from build123d import *

# Parameters (mm, degrees)
BOSS_EXTRU_1_DEPTH = 22
ESQUISSE3_W        = 22
ESQUISSE3_H        = 178
BOSS_EXTRU_2_DEPTH = 1000


with BuildPart() as part:
    # Esquisse2 → Boss.-Extru.1 (new body)
    with BuildSketch(Plane(origin=(0, 0, 0), x_dir=(1, 0, 0), z_dir=(0, 1, 0))):
        Polygon((-200, 0), (0, 0), (0, 200), (-200, 200), (-200, 105), (-100, 105), (-100, 95), (-200, 95), align=None)
    boss_extru_1 = extrude(amount=BOSS_EXTRU_1_DEPTH)

    # Symétrie1: Boss.-Extru.1 across plane
    add(boss_extru_1.mirror(Plane(origin=(0, 22, 0), x_dir=(0, 0, 1), z_dir=(-1, 0, 0))))

    # Esquisse3 → Boss.-Extru.2 (add)
    with BuildSketch(Plane(origin=(0, 22, 0), x_dir=(1, 0, 0), z_dir=(0, 1, 0))):
        Polygon((70, 200), (-70, 200), (-70, 178), (-11, 178), (11, 178), (70, 178), align=None)
        with Locations((0, 89)):
            Rectangle(ESQUISSE3_W, ESQUISSE3_H)
    extrude(amount=-BOSS_EXTRU_2_DEPTH)


solid = part.part
Part model, mm, in its own coordinate system. A direction names the side the tool comes from. Coordinates: 2 decimals unless noted, no trailing zeros. Order: outer loops, then holes, each group sorted by start corner. A loop starts at its lowest first (then second) coordinate and runs counter-clockwise, first axis right, second up.
(1) Slice it at D-D, the plane x = 54. Write the cut outline in (y, z).
Check sheet entries:
outline: (-978, -200) - (22, -200) - (22, 0) - (0, 0) - (0, -178) - (-978, -178) - close
(2) Probe L1, parallel to Z at x = -19, y = -60.5; L2, parallel to Y at x = 153.5, z = -181.5; L3, parallel to X at y = -801, z = -178.5. List the from-to ranges inside material, lowest first.
Check sheet entries:
L1: z = -200 to -178
L2: y = 0 to 22
L3: x = -70 to 70
(3) Slice it at A-A, the plane x = 121. Write the cut outline in (y, z), and give its area (3 significant figures).
Check sheet entries:
outline: (0, -200) - (22, -200) - (22, -105) - (0, -105) - close; (0, -95) - (22, -95) - (22, 0) - (0, 0) - close
area: 4,180 mm2
(4) Tool access for faces 5 (the face through (40, -482, -178)), 6 (the face through (-151, 11, -105)), 7 (the face through (-41, -482, -178)): list every direction of +Z, -Z, +X, -X, +Y, -Y with a clear straight run to the whole face (end or side of a thin tool).
Check sheet entries:
face 5: +Z, +X, -Y
face 6: -X, +Y, -Y
face 7: +Z, -X, -Y
(5) Pin check, flat tips, straight feed: pin 1 Ø11 at (y, z) = (-431.5, -188) entering from -X; pin 2 Ø1.5 at (y, z) = (-563.5, -46) entering from +X; pin 3 Ø4 at (y, z) = (-695, -93) entering from -X. Stop position of each tip, or through.
Check sheet entries:
pin 1: stops at x = -70
pin 2: stops at x = 11
pin 3: stops at x = -11
(6) Slice it at C-C, the plane y = -388. Write the cut outline in (x, z).
Check sheet entries:
outline: (-70, -200) - (70, -200) - (70, -178) - (11, -178) - (11, 0) - (-11, 0) - (-11, -178) - (-70, -178) - close
(7) Slice it at B-B, the plane z = -36.5. Write the cut outline in (x, y).
Check sheet entries:
outline: (-200, 0) - (-11, 0) - (-11, -978) - (11, -978) - (11, 0) - (200, 0) - (200, 22) - (-200, 22) - close
(8) Pull direction Z, two halves, no side cores. Call faces 1 (the face through (-149, 11, -95)), 2 (the face through (-16, -443, -200)), 3 (the face through (149, 11, -95)), 4 (the face through (-11, -482, -88)): pulls with the +Z half, pulls with the -Z half, needs draft (parallel to the pull), parting line crosses it, or undercut.
Check sheet entries:
face 1: undercut
face 2: pulls with the -Z half
face 3: undercut
face 4: needs draft
